Input: part model. Units: mm. Frame: model coordinates. Coordinates: 2 decimals unless noted, no trailing zeros. Order: outer loops, then holes, each group sorted by start corner. A loop starts at its lowest first (then second) coordinate and runs counter-clockwise, first axis right, second up. Notation, with made-up numbers: (78, 46) -> (128, 46) arc R25 cw to (128, 83) -> close; hole circle Ø1 at (0.25, 71). An arc over 180 degrees is marked (long way). Answer as CSV lines item,"result".
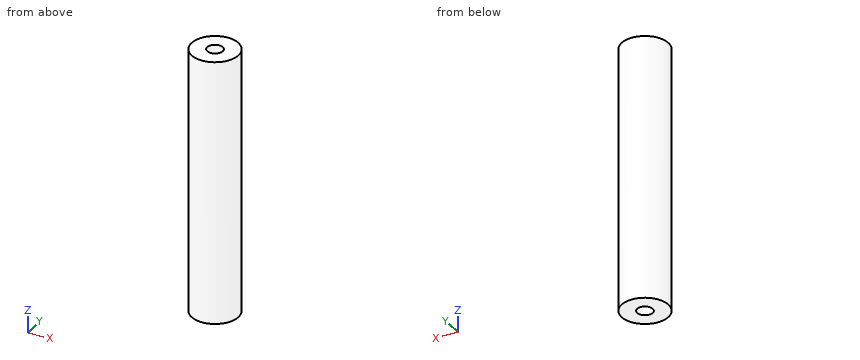
Autodesk Fusion 360 part; units mm, degrees
sketch "Sketch1" plane through (0, 0, 0) normal (0, 0, 1) x (1, 0, 0)
  circle A0 centre (0, 0) radius 4.5
  circle A1 centre (0, 0) radius 1.5
  dimension "d1" = 9
  dimension "d2" = 3
extrude "Extrude1" add sketch "Sketch1" against normal blind 50.8 contours A0 | A1
extrude "Extrude2" cut sketch "Sketch1" against normal blind 10 contours A1
sketch "Sketch2" plane through (0, 0, -50.8) normal (0, 0, -1) x (1, 0, 0)
  circle A0 centre (0, 0) radius 4.5
  circle A1 centre (0, 0) radius 1.5
extrude "Extrude3" cut sketch "Sketch2" against normal blind 10 contours A1
equation "d3 = -25.4 * 2 mm"
1. Cut plane D-D (z = -11). Return the cut outline in (x, y), plus the area to 3 significant figures.
Findings:
outline,"circle Ø9 at (0, 0)"
area,"63.6 mm2"
2. Cut plane C-C (z = -5). Return the cut outline in (x, y), plus the area to 3 significant figures.
Findings:
outline,"circle Ø9 at (0, 0); hole circle Ø3 at (0, 0)"
area,"56.5 mm2"
3. Ray query, line 1 along Y through (x, z) = (0, -3); line 2 along Z through (x, y) = (1, 0); line 3 along X through (y, z) = (-0.25, -48). Return the intervals inside material, ascending.
Findings:
line 1,"y = -4.5 to -1.5, 1.5 to 4.5"
line 2,"z = -40.8 to -10"
line 3,"x = -4.49 to -1.48, 1.48 to 4.49"
4. Cut plane A-A (y = 0). Return the cut outline in (x, z).
Findings:
outline,"(-4.5, -50.8) -> (-1.5, -50.8) -> (-1.5, -40.8) -> (1.5, -40.8) -> (1.5, -50.8) -> (4.5, -50.8) -> (4.5, 0) -> (1.5, 0) -> (1.5, -10) -> (-1.5, -10) -> (-1.5, 0) -> (-4.5, 0) -> close"
5. Contact query for flat-ended pins moving along their axis: pin 1 (2.5 mm diameter, centred on x = 0, y = 0, fed in from +Z); pin 2 (0.9 mm diameter, centred on x = 0, y = -0.5, fed in from -Z); pin 3 (1.5 mm diameter, centred on y = -2.5, z = -9.5, fed in from +X). Output: stop coordinate, or through.
Findings:
pin 1,"stops at z = -10"
pin 2,"stops at z = -40.8"
pin 3,"stops at x = 4.15"
